Verification items for the finished model (mm, model axes). A direction names the side the tool comes from. Give positions to 0.01 mm unless a question says otherwise; leave off trailing zeros. Loops run counter-clockwise (first coordinate to the right, second up) from the corner with the lowest first, then second, coordinate; pieces in that order, holes last. Notation, with made-up numbers: (13.25, 4) - (68.25, 4) arc R21 cw to (68.25, 21) - close; hole circle Ø11 at (23, 57). An arc over 180 degrees is marked (long way). One line per question, with ' | ' between items. Start each with the question number.
1. Depth check by flat-ended pin: pin 1 Ø10 at (x, y) = (-1.5, 2) entering from -Z. Enter the tip coordinate at first touch or a pass-through.
2. Mould release check, pull along X, two halves, no side actions. Record for faces 3 (the face through (18.099, -16.615, 0.345)), 4 (the face through (-19.987, -18.459, 1.232)), 5 (the face through (20.5, 0, 1)), 6 (the face through (0, 19, 1)): +X half, -X half, draft (parallel to the pull), parting line (faces both ways), or undercut.
3. Section check A-A, the plane x = -1.5. Enter the section's corners in (y, z).
4. Section check B-B, the plane y = 6.5. Enter the section's corners in (x, z).
5. Thickness scan on line 1 along X through (y, z) = (-1, 0.55); line 2 along Y through (x, z) = (-12, 0.3); line 3 along Z through (x, y) = (17, 14). Record the ranges inside material, lowest first. Write a range as from..to.
6. Tool access check on faces 1 (the face through (18.115, 16.599, 0.345)), 2 (the face through (0, -19, 1)). Record the directions out of +Z, -Z, +X, -X, +Y, -Y that give a thin tool (end or side, any length) a straight path to the whole face; none if there is none.
from build123d import *

# Parameters (mm, degrees)
FACTORY_SNAP_LID_DEPTH             = 2.5
MOULDED_LID_UNDERSIDE_RELIEF_DEPTH = 0.7


with BuildPart() as part:
    # Factory_snap_lid_Sketch → Factory_snap_lid (new body)
    with BuildSketch(Plane.XY):
        with BuildLine():
            Line((-18.7, -19), (18.7, -19))
            ThreePointArc((18.7, -19), (19.972792206, -18.472792206), (20.5, -17.2))
            Line((20.5, -17.2), (20.5, 17.2))
            ThreePointArc((20.5, 17.2), (19.972792206, 18.472792206), (18.7, 19))
            Line((18.7, 19), (-18.7, 19))
            ThreePointArc((-18.7, 19), (-19.972792206, 18.472792206), (-20.5, 17.2))
            Line((-20.5, 17.2), (-20.5, -17.2))
            ThreePointArc((-20.5, -17.2), (-19.972792206, -18.472792206), (-18.7, -19))
        make_face()
    extrude(amount=FACTORY_SNAP_LID_DEPTH)

    # Moulded_lid_underside_relief_Sketch → Moulded_lid_underside_relief (cut)
    with BuildSketch(Plane.XY):
        with BuildLine():
            Line((-17.4, -16.9), (17.4, -16.9))
            ThreePointArc((17.4, -16.9), (18.107106781, -16.607106781), (18.4, -15.9))
            Line((18.4, -15.9), (18.4, 15.9))
            ThreePointArc((18.4, 15.9), (18.107106781, 16.607106781), (17.4, 16.9))
            Line((17.4, 16.9), (-17.4, 16.9))
            ThreePointArc((-17.4, 16.9), (-18.107106781, 16.607106781), (-18.4, 15.9))
            Line((-18.4, 15.9), (-18.4, -15.9))
            ThreePointArc((-18.4, -15.9), (-18.107106781, -16.607106781), (-17.4, -16.9))
        make_face()
    extrude(amount=MOULDED_LID_UNDERSIDE_RELIEF_DEPTH, mode=Mode.SUBTRACT)


solid = part.part
Results list:
1) pin 1: z = 0.7
2) face 3: undercut | face 4: -X half | face 5: +X half | face 6: draft
3) outline: (-19, 0) - (-16.9, 0) - (-16.9, 0.7) - (16.9, 0.7) - (16.9, 0) - (19, 0) - (19, 2.5) - (-19, 2.5) - close
4) outline: (-20.5, 0) - (-18.4, 0) - (-18.4, 0.7) - (18.4, 0.7) - (18.4, 0) - (20.5, 0) - (20.5, 2.5) - (-20.5, 2.5) - close
5) line 1: -20.5..-18.4, 18.4..20.5 | line 2: -19..-16.9, 16.9..19 | line 3: 0.7..2.5
6) face 1: -Z | face 2: +Z, -Z, +X, -X, -Y
